Here's the drawing with two shaded views (mm, measured from the low corner). I have some questions. Coordinates: 2 decimals unless noted, no trailing zeros. Order: outer loops, then holes, each group sorted by start corner. A loop starts at its lowest first (then second) coordinate and runs counter-clockwise, first axis right, second up. Notation, with made-up numbers: (58, 42) - (104, 42) arc R21 cw to (104, 73) - close; hole circle Ø10 at (17.5, 27.5). An arc over 180 degrees is marked (long way). One line per item, written item: value. Start each with the question number.
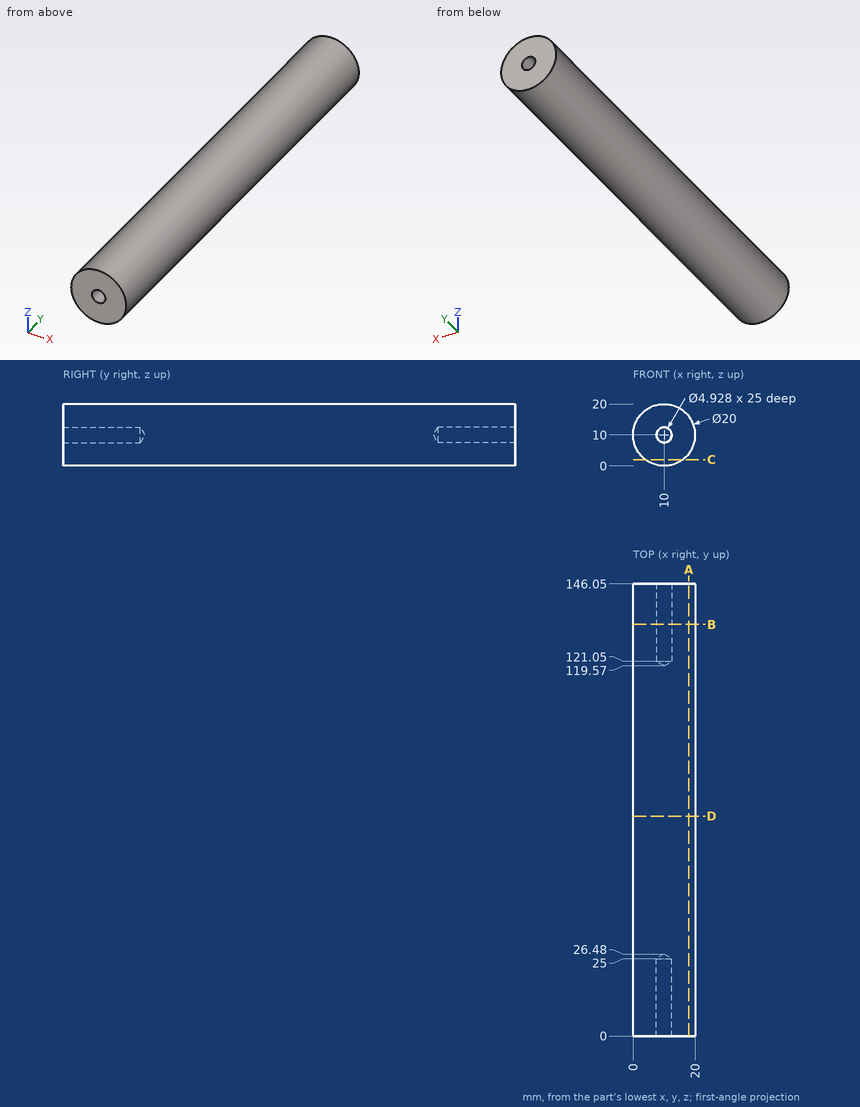
Q1. If I drill on L1, parallel to Z at x = 10, y = 128; L2, parallel to Z at x = 6.5, y = 16; L3, parallel to Z at x = 16.75, y = 68.5, over which ranges is the centre line in solid material (lowest first)?
Q2. I want a section at A-A on x = 18. Please give me the cut outline in (y, z).
Q3. I want a section at B-B on y = 133. Please give me the cut outline in (x, z), then the cut area to 3 significant figures.
Q4. I'm going to push flat-ended pins straight in: pin 1 (1 mm diameter, centred on x = 11.5, y = 76.5, fed in from -Z); pin 2 (3 mm diameter, centred on y = 35.5, z = 13, fed in from +X); pin 3 (1 mm diameter, centred on y = 104.5, z = 7, fed in from -X). Where does each tip first touch, or does it pass through?
Q5. I want a section at C-C on z = 2. Please give me the cut outline in (x, y), then the cut area to 3 significant figures.
Q6. I want a section at D-D on y = 71. Please give me the cut outline in (x, z).
Values follow:
1. L1: z = 0 to 7.54, 12.46 to 20
1. L2: z = 0.63 to 19.37
1. L3: z = 2.62 to 17.38
2. outline: (0, 4) - (146.05, 4) - (146.05, 16) - (0, 16) - close
3. outline: circle Ø20 at (10, 10); hole circle Ø4.93 at (10, 10)
3. area: 295 mm^2
4. pin 1: stops at z = 0.05
4. pin 2: stops at x = 19.89
4. pin 3: stops at x = 0.32
5. outline: (4, 0) - (16, 0) - (16, 146.05) - (4, 146.05) - close
5. area: 1,750 mm^2
6. outline: circle Ø20 at (10, 10)
